```python
from build123d import *

# Parameters (mm, degrees)
F1_DEPTH = 3.175
F2_R     = 1.5875


with BuildPart() as f1:
    # F0 (on Top) → F1 (new body)
    with BuildSketch(Plane.XY):
        Polygon((-15.875, -24.60625), (-12.7, -24.60625), (-12.7, -24.463631), (-12.7, -22.876131), (-12.7, -21.298139), (-12.7, -19.710639), (-12.7, -18.132646), (-12.7, -16.545146), (-12.7, -14.967154), (-12.7, -13.379654), (-12.7, -11.801662), (-12.7, -10.214162), (-12.7, -8.63617), (-12.7, -7.04867), (-12.7, -5.470678), (-12.7, -3.883178), (-12.7, -2.305186), (-12.7, -0.717686), (-12.7, 0.860306), (-12.7, 2.447806), (-12.7, 4.025798), (-12.7, 5.613298), (-12.7, 7.19129), (-12.7, 8.77879), (-12.7, 10.356782), (-12.7, 11.944282), (-12.7, 13.522274), (-12.7, 15.109774), (-12.7, 16.687766), (-12.7, 18.275266), (-12.7, 19.853258), (-12.7, 21.440758), (-12.7, 23.01875), (-12.7, 24.60625), (-15.875, 24.60625), align=None)
        with BuildLine():
            Line((-12.7, -22.876131), (-12.7, -24.463631))
            Line((-12.7, -24.463631), (-11.90625, -24.463631))
            ThreePointArc((-11.90625, -24.463631), (-11.344984, -24.231147), (-11.1125, -23.669881))
            ThreePointArc((-11.1125, -23.669881), (-11.344984, -23.108615), (-11.90625, -22.876131))
            Line((-11.90625, -22.876131), (-12.7, -22.876131))
        make_face()
        with BuildLine():
            Line((-12.7, -19.710639), (-12.7, -21.298139))
            Line((-12.7, -21.298139), (-11.90625, -21.298139))
            ThreePointArc((-11.90625, -21.298139), (-11.344984, -21.065655), (-11.1125, -20.504389))
            ThreePointArc((-11.1125, -20.504389), (-11.344984, -19.943123), (-11.90625, -19.710639))
            Line((-11.90625, -19.710639), (-12.7, -19.710639))
        make_face()
        with BuildLine():
            Line((-12.7, -16.545146), (-12.7, -18.132646))
            Line((-12.7, -18.132646), (-11.90625, -18.132646))
            ThreePointArc((-11.90625, -18.132646), (-11.344984, -17.900162), (-11.1125, -17.338896))
            ThreePointArc((-11.1125, -17.338896), (-11.344984, -16.77763), (-11.90625, -16.545146))
            Line((-11.90625, -16.545146), (-12.7, -16.545146))
        make_face()
        with BuildLine():
            Line((-12.7, -13.379654), (-12.7, -14.967154))
            Line((-12.7, -14.967154), (-11.90625, -14.967154))
            ThreePointArc((-11.90625, -14.967154), (-11.344984, -14.73467), (-11.1125, -14.173404))
            ThreePointArc((-11.1125, -14.173404), (-11.344984, -13.612138), (-11.90625, -13.379654))
            Line((-11.90625, -13.379654), (-12.7, -13.379654))
        make_face()
        with BuildLine():
            Line((-12.7, -10.214162), (-12.7, -11.801662))
            Line((-12.7, -11.801662), (-11.90625, -11.801662))
            ThreePointArc((-11.90625, -11.801662), (-11.344984, -11.569178), (-11.1125, -11.007912))
            ThreePointArc((-11.1125, -11.007912), (-11.344984, -10.446646), (-11.90625, -10.214162))
            Line((-11.90625, -10.214162), (-12.7, -10.214162))
        make_face()
        with BuildLine():
            Line((-12.7, -7.04867), (-12.7, -8.63617))
            Line((-12.7, -8.63617), (-11.90625, -8.63617))
            ThreePointArc((-11.90625, -8.63617), (-11.344984, -8.403686), (-11.1125, -7.84242))
            ThreePointArc((-11.1125, -7.84242), (-11.344984, -7.281154), (-11.90625, -7.04867))
            Line((-11.90625, -7.04867), (-12.7, -7.04867))
        make_face()
        with BuildLine():
            Line((-12.7, -3.883178), (-12.7, -5.470678))
            Line((-12.7, -5.470678), (-11.90625, -5.470678))
            ThreePointArc((-11.90625, -5.470678), (-11.344984, -5.238194), (-11.1125, -4.676928))
            ThreePointArc((-11.1125, -4.676928), (-11.344984, -4.115662), (-11.90625, -3.883178))
            Line((-11.90625, -3.883178), (-12.7, -3.883178))
        make_face()
        with BuildLine():
            Line((-12.7, -0.717686), (-12.7, -2.305186))
            Line((-12.7, -2.305186), (-11.90625, -2.305186))
            ThreePointArc((-11.90625, -2.305186), (-11.344984, -2.072702), (-11.1125, -1.511436))
            ThreePointArc((-11.1125, -1.511436), (-11.344984, -0.95017), (-11.90625, -0.717686))
            Line((-11.90625, -0.717686), (-12.7, -0.717686))
        make_face()
        with BuildLine():
            Line((-11.90625, 2.447806), (-12.7, 2.447806))
            Line((-12.7, 2.447806), (-12.7, 0.860306))
            Line((-12.7, 0.860306), (-11.90625, 0.860306))
            ThreePointArc((-11.90625, 0.860306), (-11.344984, 1.09279), (-11.1125, 1.654056))
            ThreePointArc((-11.1125, 1.654056), (-11.344984, 2.215322), (-11.90625, 2.447806))
        make_face()
        with BuildLine():
            Line((-11.90625, 5.613298), (-12.7, 5.613298))
            Line((-12.7, 5.613298), (-12.7, 4.025798))
            Line((-12.7, 4.025798), (-11.90625, 4.025798))
            ThreePointArc((-11.90625, 4.025798), (-11.344984, 4.258282), (-11.1125, 4.819548))
            ThreePointArc((-11.1125, 4.819548), (-11.344984, 5.380814), (-11.90625, 5.613298))
        make_face()
        with BuildLine():
            Line((-11.90625, 8.77879), (-12.7, 8.77879))
            Line((-12.7, 8.77879), (-12.7, 7.19129))
            Line((-12.7, 7.19129), (-11.90625, 7.19129))
            ThreePointArc((-11.90625, 7.19129), (-11.344984, 7.423774), (-11.1125, 7.98504))
            ThreePointArc((-11.1125, 7.98504), (-11.344984, 8.546306), (-11.90625, 8.77879))
        make_face()
        with BuildLine():
            Line((-11.90625, 11.944282), (-12.7, 11.944282))
            Line((-12.7, 11.944282), (-12.7, 10.356782))
            Line((-12.7, 10.356782), (-11.90625, 10.356782))
            ThreePointArc((-11.90625, 10.356782), (-11.344984, 10.589266), (-11.1125, 11.150532))
            ThreePointArc((-11.1125, 11.150532), (-11.344984, 11.711798), (-11.90625, 11.944282))
        make_face()
        with BuildLine():
            Line((-11.90625, 15.109774), (-12.7, 15.109774))
            Line((-12.7, 15.109774), (-12.7, 13.522274))
            Line((-12.7, 13.522274), (-11.90625, 13.522274))
            ThreePointArc((-11.90625, 13.522274), (-11.344984, 13.754758), (-11.1125, 14.316024))
            ThreePointArc((-11.1125, 14.316024), (-11.344984, 14.87729), (-11.90625, 15.109774))
        make_face()
        with BuildLine():
            Line((-11.90625, 18.275266), (-12.7, 18.275266))
            Line((-12.7, 18.275266), (-12.7, 16.687766))
            Line((-12.7, 16.687766), (-11.90625, 16.687766))
            ThreePointArc((-11.90625, 16.687766), (-11.344984, 16.92025), (-11.1125, 17.481516))
            ThreePointArc((-11.1125, 17.481516), (-11.344984, 18.042782), (-11.90625, 18.275266))
        make_face()
        with BuildLine():
            Line((-11.90625, 21.440758), (-12.7, 21.440758))
            Line((-12.7, 21.440758), (-12.7, 19.853258))
            Line((-12.7, 19.853258), (-11.90625, 19.853258))
            ThreePointArc((-11.90625, 19.853258), (-11.344984, 20.085742), (-11.1125, 20.647008))
            ThreePointArc((-11.1125, 20.647008), (-11.344984, 21.208274), (-11.90625, 21.440758))
        make_face()
        with BuildLine():
            Line((-11.90625, 24.60625), (-12.7, 24.60625))
            Line((-12.7, 24.60625), (-12.7, 23.01875))
            Line((-12.7, 23.01875), (-11.90625, 23.01875))
            ThreePointArc((-11.90625, 23.01875), (-11.344984, 23.251234), (-11.1125, 23.8125))
            ThreePointArc((-11.1125, 23.8125), (-11.344984, 24.373766), (-11.90625, 24.60625))
        make_face()
    extrude(amount=F1_DEPTH)

    # F2
    f2_edges = [f1.edges().sort_by_distance(p)[0] for p in [
        (-15.875, 24.60625, 1.5875),
        (-15.875, -24.60625, 1.5875),
    ]]
    fillet(f2_edges, radius=F2_R)


solid = f1.part
```
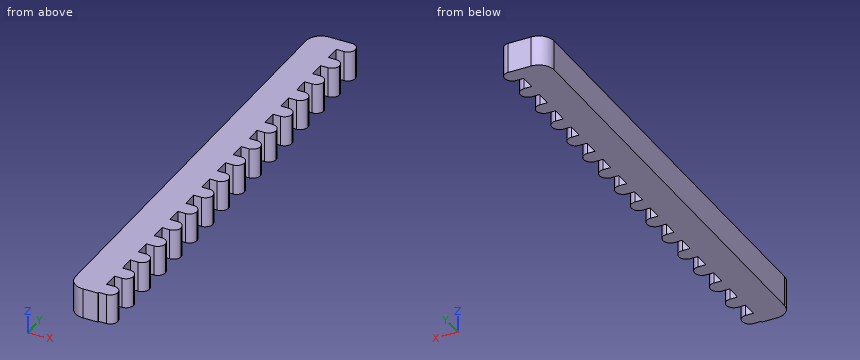
Input: part model. Units: mm. Frame: model coordinates. Coordinates: 2 decimals unless noted, no trailing zeros. Order: outer loops, then holes, each group sorted by start corner. A loop starts at its lowest first (then second) coordinate and runs counter-clockwise, first axis right, second up. Notation, with made-up numbers: (22, 68) - (53, 68) arc R22 ccw to (53, 74) - close; hole circle Ø8 at (45, 60). An arc over 180 degrees is marked (long way). Put each result on its own line as item: value.
1. Contact query for flat-ended pins moving along their axis: pin 1 Ø0.6 at (x, z) = (-12, 1.5) entering from -Y; pin 2 Ø0.9 at (x, z) = (-12.5, 1) entering from -Y; pin 3 Ø0.8 at (y, z) = (-16, 1) entering from +X; pin 4 Ø1.5 at (y, z) = (9, 1.5) entering from +X. Output: stop coordinate, or through.
Report:
pin 1: stops at y = -24.46
pin 2: stops at y = -24.61
pin 3: stops at x = -12.7
pin 4: stops at x = -11.16
2. Line query: line 1 along X through (y, z) = (-6, 2.55) (3 decimals); line 2 along Y through (x, z) = (-14.45, 2.9); line 3 along X through (y, z) = (-14, 1.1) (3 decimals). Output: solid intervals per line, ascending.
Report:
line 1: x = -15.875 to -12.7
line 2: y = -24.6 to 24.6
line 3: x = -15.875 to -11.132
3. Cut plane A-A on y = 3. Return the cut outline in (x, z) (3 decimals), then the cut area to 3 significant figures.
Report:
outline: (-15.875, 0) - (-12.7, 0) - (-12.7, 3.175) - (-15.875, 3.175) - close
area: 10.1 mm2
